Solid Edge part; units mm, degrees
sketch "Sketch1" plane through (0, 0, 0) normal (0, 0, 1) x (1, 0, 0)
  line L0 (5.7895, 6.6667) -> (5.7895, 36.6667)
  line L1 (5.7895, 36.6667) -> (65.7895, 36.6667)
  line L2 (65.7895, 36.6667) -> (65.7895, 6.6667)
  line L3 (65.7895, 6.6667) -> (5.7895, 6.6667)
  dimension "D1" = 5.7895
  dimension "D2" = 5.7895
extrude "Protrusion1" add sketch "Sketch1" along normal blind 8
fillet "Round_1" radius 5 2 edges at (65.7895, 36.6667, 4) (5.7895, 36.6667, 4)
sketch "Sketch2" plane through (35.7895, 21.6667, 8) normal (0, 0, 1) x (0, 1, 0)
  line L0 (-15, 10) -> (-11, 10)
  line L1 (-11, 10) -> (-11, -10)
  line L2 (-11, -10) -> (-15, -10)
  line L3 (-15, -10) -> (-15, 10)
  dimension "D1" = 11
extrude "ExtrudedProtrusion_3" add sketch "Sketch2" along normal blind 80
sketch "Sketch3" plane through (35.7895, 10.6667, 48) normal (0, 1, 0) x (0, 0, -1)
  circle A0 centre (-40.1226, 0) radius 10.0008
extrude "ExtrudedProtrusion_4" add sketch "Sketch3" against normal blind 13
fillet "Round_4" radius 10 2 edges at (45.7895, 8.6667, 8) (25.7895, 8.6667, 8)
sketch "Sketch4" plane through (35.7895, -2.3333, 88.1226) normal (0, -1, 0) x (1, 0, 0)
  circle A0 centre (0, 0) radius 7.9922
extrude "Cutout1" cut sketch "Sketch4" against normal through all
Input: part model. Units: mm. Frame: model coordinates. A direction names the side the tool comes from. Coordinates: 2 decimals unless noted, no trailing zeros. Loops run counter-clockwise (first coordinate to the right, second up) from the corner with the lowest first, then second, coordinate; pieces in that order, holes last. Notation, with made-up numbers: (-37.75, 89) -> (3.25, 89) arc R19 cw to (3.25, 109) -> close; hole circle Ø8 at (44.25, 24). An arc over 180 degrees is marked (long way). Use a Markdown table: item, result.
1) Cut plane A-A (x = 29). Return the cut outline in (y, z).
Results found:
| item | result |
|---|---|
| outline | (-2.33, 80.78) -> (6.67, 80.78) -> (6.67, 0) -> (36.67, 0) -> (36.67, 8) -> (10.67, 8) -> (10.67, 83.91) -> (-2.33, 83.91) -> close; (-2.33, 92.34) -> (10.67, 92.34) -> (10.67, 95.47) -> (-2.33, 95.47) -> close |
2) Cut plane D-D (z = 39.5). Return the cut outline in (x, y).
Results found:
| item | result |
|---|---|
| outline | (25.79, 6.67) -> (45.79, 6.67) -> (45.79, 10.67) -> (25.79, 10.67) -> close |
3) Cut plane C-C (x = 51.5). Return the cut outline in (y, z), then the cut area to 3 significant figures.
Results found:
| item | result |
|---|---|
| outline | (6.67, 0) -> (36.67, 0) -> (36.67, 8) -> (10.67, 8) -> (10.67, 8.97) -> (6.67, 8.97) -> close |
| area | 244 mm2 |
4) Pull-direction query (Z, two-part tool) for faces 4 (the flat face through (65.79, 19, 4)), 5 (the flat face through (36, 22, 8)), 6 (the cylindrical face through (35.35, 2.813, 98.114)), 7 (the cylindrical face through (34.06, 4.08, 80.32)); classes: released by +Z, released by -Z, zero draft, split by the parting line, or undercut.
Results found:
| item | result |
|---|---|
| face 4 | zero draft |
| face 5 | released by +Z |
| face 6 | split by the parting line |
| face 7 | undercut |
5) Contact query for flat-ended pins moving along their axis: pin 1 (12 mm diameter, centred on y = 14, z = 32, fed in from +X); pin 2 (4 mm diameter, centred on x = 27, y = 17, fed in from +Z); pin 3 (8 mm diameter, centred on x = 24, z = 12.5, fed in from -Y). Output: stop coordinate, or through.
Results found:
| item | result |
|---|---|
| pin 1 | stops at x = 45.79 |
| pin 2 | stops at z = 8 |
| pin 3 | stops at y = 6.67 |
6) Material intervals for line 1 along Z through (x, y) = (23.5, 35.5); line 2 along Z through (x, y) = (39, 5.5); line 3 along Y through (x, z) = (28, 85.5), sorted ascending. Write a range as from..to.
Results found:
| item | result |
|---|---|
| line 1 | z = 0..8 |
| line 2 | z = 78.65..80.8, 95.44..97.59 |
| line 3 | y = -2.33..10.67 |
7) Cut plane B-B (y = 26.5). Return the cut outline in (x, z).
Results found:
| item | result |
|---|---|
| outline | (5.79, 0) -> (65.79, 0) -> (65.79, 8) -> (5.79, 8) -> close |
8) Access query for faces 1 (the flat face through (45.79, 9, 53)), 2 (the flat face through (25.79, 9, 53)), 3 (the flat face through (36, 10.667, 42)). Directions: +Z, -Z, +X, -X, +Y, -Y. A direction counts if a zero-diameter tool reaches every point of the face in a straight line with its end or side. Return the directions, or none.
Results found:
| item | result |
|---|---|
| face 1 | +Z, +X, +Y, -Y |
| face 2 | +Z, -X, +Y, -Y |
| face 3 | +Z, +X, -X, +Y |
